```python
from build123d import *

# Parameters (mm, degrees)
ESQUISSE1_R               = 50
BOSS_EXTRU_1_DEPTH        = 1.6
ENL_V_MAT_EXTRU_1_DEPTH   = 1.6
ESQUISSE4_R               = 12
ENL_V_MAT_EXTRU_3_DEPTH   = 1.6
ESQUISSE7_R               = 1
ENL_V_MAT_EXTRU_4_DEPTH   = 1.6
SYM_TRIE8_COPY_1_SKETCH_R = 1
SYM_TRIE8_COPY_1_DEPTH    = 1.6


with BuildPart() as part:
    # Esquisse1 → Boss.-Extru.1 (new body)
    with BuildSketch(Plane.XY):
        Circle(ESQUISSE1_R)
    extrude(amount=BOSS_EXTRU_1_DEPTH)

    # Esquisse2 → Enlèv. mat.-Extru.1 (cut)
    with BuildSketch(Plane.XY.offset(1.6)):
        with BuildLine():
            Line((-33.5, 15), (-33.5, -15))
            ThreePointArc((-33.5, -15), (-39, -20.5), (-44.5, -15))
            Line((-44.5, -15), (-44.5, 15))
            ThreePointArc((-44.5, 15), (-39, 20.5), (-33.5, 15))
        make_face()
    enl_v_mat_extru_1 = extrude(amount=-ENL_V_MAT_EXTRU_1_DEPTH, mode=Mode.SUBTRACT)

    # Symétrie1: Enlèv. mat.-Extru.1 across plane
    add(enl_v_mat_extru_1.mirror(Plane(origin=(0, 0, 0), x_dir=(0, 0, 1), z_dir=(1, 0, 0))), mode=Mode.SUBTRACT)

    # Esquisse4 → Enlèv. mat.-Extru.3 (cut)
    with BuildSketch(Plane.XY.offset(1.6)):
        with Locations((0, 34)):
            Circle(ESQUISSE4_R)
    enl_v_mat_extru_3 = extrude(amount=-ENL_V_MAT_EXTRU_3_DEPTH, mode=Mode.SUBTRACT)

    # Symétrie6: Enlèv. mat.-Extru.3 across plane
    add(enl_v_mat_extru_3.mirror(Plane.ZX), mode=Mode.SUBTRACT)

    # Esquisse7 → Enlèv. mat.-Extru.4 (cut)
    with BuildSketch(Plane.XY.offset(1.6)):
        with Locations((25.25, -9.221094574)):
            Circle(ESQUISSE7_R)
    enl_v_mat_extru_4 = extrude(amount=-ENL_V_MAT_EXTRU_4_DEPTH, mode=Mode.SUBTRACT)

    # Symétrie7: Enlèv. mat.-Extru.4 across plane
    add(enl_v_mat_extru_4.mirror(Plane.ZX), mode=Mode.SUBTRACT)

    # Symétrie8: Enlèv. mat.-Extru.4 across plane
    add(enl_v_mat_extru_4.mirror(Plane(origin=(0, 0, 0), x_dir=(0, 0, 1), z_dir=(1, 0, 0))), mode=Mode.SUBTRACT)

    # Symétrie8 copy 1 sketch → Symétrie8 copy 1 (cut)
    with BuildSketch(Plane(origin=(0, 0, 1.6), x_dir=(-1, 0, 0), z_dir=(0, 0, 1))):
        with Locations((25.25, -9.221094574)):
            Circle(SYM_TRIE8_COPY_1_SKETCH_R)
    extrude(amount=-SYM_TRIE8_COPY_1_DEPTH, mode=Mode.SUBTRACT)


solid = part.part
```
CAD build for the part. Positions are in the model's coordinates, mm. A direction names the side the tool comes from. Give positions to 0.01 mm unless a question says otherwise; leave off trailing zeros. Loops run counter-clockwise (first coordinate to the right, second up) from the corner with the lowest first, then second, coordinate; pieces in that order, holes last. Notation, with made-up numbers: (70.25, 88.5) - (96.25, 88.5) arc R14 ccw to (96.25, 102.5) - close; hole circle Ø11 at (-27.75, 18). An arc over 180 degrees is marked (long way). Put each result on its own line as item: value.
Q1. Slice it at D-D (x = -39). Give the cut face in (y, z), plus the area to 3 significant figures.
Filled in:
outline: (-31.29, 0) - (-20.5, 0) - (-20.5, 1.6) - (-31.29, 1.6) - close; (20.5, 0) - (31.29, 0) - (31.29, 1.6) - (20.5, 1.6) - close
area: 34.5 mm²
Q2. Flat gauge pins, fed straight in: pin 1 (0.8 mm diameter, centred on y = 3, z = 0.5, fed in from +X); pin 2 (2.5 mm diameter, centred on x = -25.25, y = 9.22, fed in from -Z); pin 3 (0.5 mm diameter, centred on y = -4.5, z = 1, fed in from +X). Where does each tip first touch, or does it go through?
Filled in:
pin 1: stops at x = 49.93
pin 2: stops at z = 0
pin 3: stops at x = 49.82
Q3. Slice it at B-B (x = 0). Give the cut face in (y, z), plus the area to 3 significant figures.
Filled in:
outline: (-50, 0) - (-46, 0) - (-46, 1.6) - (-50, 1.6) - close; (-22, 0) - (22, 0) - (22, 1.6) - (-22, 1.6) - close; (46, 0) - (50, 0) - (50, 1.6) - (46, 1.6) - close
area: 83.2 mm²
Q4. Slice it at A-A (y = 0). Give the cut face in (x, z), plus the area to 3 significant figures.
Filled in:
outline: (-50, 0) - (-44.5, 0) - (-44.5, 1.6) - (-50, 1.6) - close; (-33.5, 0) - (33.5, 0) - (33.5, 1.6) - (-33.5, 1.6) - close; (44.5, 0) - (50, 0) - (50, 1.6) - (44.5, 1.6) - close
area: 125 mm²
Q5. Tool access for faces 4 (the face through (38.9, -20.5, 0.8)), 5 (the face through (-1, 1, 1.6)): list every direction of +Z, -Z, +X, -X, +Y, -Y with a clear straight run to the whole face (end or side of a thin tool).
Filled in:
face 4: +Z, -Z
face 5: +Z, +X, -X, +Y, -Y
Q6. Probe line 1 along Y through (x, z) = (0, 1.2); line 2 along Y through (x, z) = (-25.25, 1.25); line 3 along X through (y, z) = (-17, 1.55). List the from-to ranges inside material, lowest first.
Filled in:
line 1: y = -50 to -46, -22 to 22, 46 to 50
line 2: y = -43.16 to -10.22, -8.22 to 8.22, 10.22 to 43.16
line 3: x = -47.02 to -44.12, -33.88 to 33.88, 44.12 to 47.02
Q7. Slice it at C-C (y = 42). Give the cut face in (x, z).
Filled in:
outline: (-27.13, 0) - (-8.94, 0) - (-8.94, 1.6) - (-27.13, 1.6) - close; (8.94, 0) - (27.13, 0) - (27.13, 1.6) - (8.94, 1.6) - close
Q8. Mould opens along Y. For faces 1 (the face through (-1, 1, 0)), 2 (the face through (-11.99, -34.53, 0.81)), 3 (the face through (47.69, 15.02, 0.79)) say: pulls with the +Y half, pulls with the -Y half, needs draft (parallel to the pull), parting line crosses it, or undercut.
Filled in:
face 1: needs draft
face 2: undercut
face 3: parting line crosses it
